The listing builds one solid part. Answer for the finished solid, in the listing's coordinates (mm). Face numbers are marked on the shaded views. A direction names the side the tool comes from. Give positions to 0.01 mm unless a question says otherwise; leave off trailing zeros. Write each loop counter-clockwise with the first axis right and the second up, starting at its lowest first coordinate (ties: lowest second). Pieces come first, ordered by that corner, then holes. Notation, with made-up numbers: (60.25, 70.25) -> (108.25, 70.25) arc R20 ccw to (108.25, 96.25) -> close; hole circle Ø6 at (71, 44). An arc over 180 degrees is marked (long way). Put each result on its own line as item: value. Start each with the question number.
1) A cutting plane is placed at C-C (x = 20.5). Write down the section's boundary in (y, z).
2) A cutting plane is placed at B-B (y = -9.5). Write down the section's boundary in (x, z).
3) For a pull along X with two mould halves and no side action, classify the marked faces 1, 2 and 3 as released by +X, released by -X, zero draft, split by the parting line, or undercut.
4) A cutting plane is placed at A-A (z = -29). Write down the section's boundary in (x, y) (3 decimals).
5) Flat-ended cylindrical pins translate along their axes: pin 1 Ø1 at (x, y) = (14.5, 0.5) entering from -Z; pin 2 Ø1.6 at (x, z) = (15.5, -4) entering from -Y; pin 3 Ø1 at (x, y) = (7, 3) entering from -Z; pin 4 Ø5 at (x, y) = (15.625, -10.5) entering from -Z. Find the tip coordinate at first contact, or state that the pin passes through.
6) Find the intervals of material crossed by line 1 along X through (y, z) = (-10.5, -18.5); line 2 along Z through (x, y) = (11, -3.5), in increasing order. Write a range as from..to.
7) For the marked faces 4 and 5, determine the directions among +Z, -Z, +X, -X, +Y, -Y from which every point of the face is accessible in a straight line to the end or side of a thin tool.
8) A cutting plane is placed at D-D (z = -7.5). Write down the section's boundary in (x, y) (3 decimals).
from build123d import *

# Parameters (mm, degrees)
BOSS_EXTRUDE1_DEPTH = 2
SKETCH3_R           = 0.85
BOSS_EXTRUDE2_DEPTH = 8
SKETCH4_W           = 31.25
SKETCH4_H           = 3
BOSS_EXTRUDE3_DEPTH = 18
SKETCH12_R          = 2.075
CUT_EXTRUDE2_DEPTH  = 58.667690261
RIB1_REACH          = 59.668
SKETCH13_WALL_W     = 148.141224122
SKETCH13_WALL_H     = 4
RIB2_REACH          = 59.668
SKETCH14_WALL_W     = 148.141224122
SKETCH14_WALL_H     = 4


with BuildPart() as part:
    # Sketch2 → Boss-Extrude1 (new body)
    with BuildSketch(Plane(origin=(0, 0, 0), x_dir=(1, 0, 0), z_dir=(0, 1, 0))):
        Polygon((0, 0), (0, 45), (7.125, 45), (7.125, 21), (24.125, 21), (24.125, 45), (31.25, 45), (31.25, 0), align=None)
    extrude(amount=BOSS_EXTRUDE1_DEPTH)

    # Sketch3 → Boss-Extrude2 (add)
    with BuildSketch(Plane(origin=(0, 2, 0), x_dir=(1, 0, 0), z_dir=(0, 1, 0))):
        with Locations(Location((5.125, 43, 0), (0, 0, 90))):
            Circle(SKETCH3_R)
        with Locations(Location((5.125, 30.5, 0), (0, 0, 90))):
            Circle(SKETCH3_R)
        with Locations(Location((26.125, 30.5, 0), (0, 0, 90))):
            Circle(SKETCH3_R)
        with Locations(Location((26.125, 43, 0), (0, 0, 90))):
            Circle(SKETCH3_R)
    extrude(amount=BOSS_EXTRUDE2_DEPTH)

    # Sketch4 → Boss-Extrude3 (add)
    with BuildSketch(Plane.XZ):
        with Locations((15.625, -1.5)):
            Rectangle(SKETCH4_W, SKETCH4_H)
        with Locations((15.625, -7.75)):
            Rectangle(SKETCH4_W, SKETCH4_H)
    extrude(amount=BOSS_EXTRUDE3_DEPTH)

    # Sketch12 → Cut-Extrude2 (cut, through all)
    with BuildSketch(Plane.XY):
        with Locations((15.625, -10.5)):
            Circle(SKETCH12_R)
    extrude(amount=-CUT_EXTRUDE2_DEPTH, mode=Mode.SUBTRACT)

    # Sketch13 wall → Rib1 (add, up to next)
    with BuildSketch(Plane(origin=(0, -9, -21.75), x_dir=(0, -0.584304725845, 0.811534341451), z_dir=(0, -0.811534341451, -0.584304725845)), mode=Mode.PRIVATE) as rib1_sk1:
        with Locations((0, -2)):
            Rectangle(SKETCH13_WALL_W, SKETCH13_WALL_H)
    rib1_tool1 = extrude(rib1_sk1.sketch, amount=-RIB1_REACH, mode=Mode.PRIVATE) - part.part
    add(rib1_tool1.solids().sort_by_distance((0, -9, -21.75))[0])

    # Sketch14 wall → Rib2 (add, up to next)
    with BuildSketch(Plane(origin=(31.25, -9, -21.75), x_dir=(0, -0.584304725845, 0.811534341451), z_dir=(0, -0.811534341451, -0.584304725845)), mode=Mode.PRIVATE) as rib2_sk1:
        with Locations((0, 2)):
            Rectangle(SKETCH14_WALL_W, SKETCH14_WALL_H)
    rib2_tool1 = extrude(rib2_sk1.sketch, amount=-RIB2_REACH, mode=Mode.PRIVATE) - part.part
    add(rib2_tool1.solids().sort_by_distance((31.25, -9, -21.75))[0])


solid = part.part
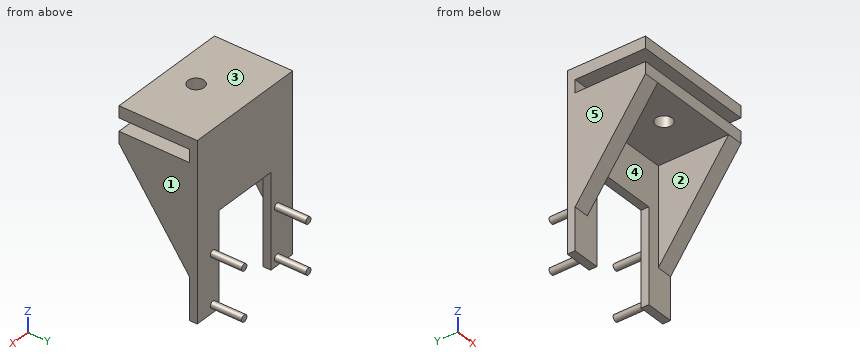
Reply:
1. outline: (-18, -9.25) -> (0, -9.25) -> (0, -21) -> (2, -21) -> (2, 0) -> (-18, 0) -> (-18, -3) -> (0, -3) -> (0, -6.25) -> (-18, -6.25) -> close
2. outline: (0, -21.06) -> (4, -21.06) -> (4, -9.25) -> (13.81, -9.25) -> (13.81, -6.25) -> (0, -6.25) -> close; (0, -3) -> (13.81, -3) -> (13.81, 0) -> (0, 0) -> close; (17.44, -9.25) -> (27.25, -9.25) -> (27.25, -21.06) -> (31.25, -21.06) -> (31.25, -6.25) -> (17.44, -6.25) -> close; (17.44, -3) -> (31.25, -3) -> (31.25, 0) -> (17.44, 0) -> close
3. face 1: released by +X
3. face 2: undercut
3. face 3: zero draft
4. outline: (0, -3.78) -> (4, -3.78) -> (4, 0) -> (7.125, 0) -> (7.125, 2) -> (0, 2) -> close; (24.125, 0) -> (27.25, 0) -> (27.25, -3.78) -> (31.25, -3.78) -> (31.25, 2) -> (24.125, 2) -> close
5. pin 1: stops at z = -21
5. pin 2: stops at y = 0
5. pin 3: passes through
5. pin 4: stops at z = -9.25
6. line 1: x = 0..4, 27.25..31.25
6. line 2: z = -9.25..-6.25, -3..0
7. face 4: -Z, -Y
7. face 5: +Z, -Z, -X, +Y, -Y
8. outline: (0, -18) -> (31.25, -18) -> (31.25, 2) -> (0, 2) -> close; hole circle Ø4.15 at (15.625, -10.5)
